For this review, take the finished solid that the model builds, in its own axes (mm). Face numbers are marked on the shaded views. A direction names the side the tool comes from. Give positions to 0.01 mm unless a question says otherwise; leave off trailing zeros. Order: outer loops, then holes, each group sorted by start corner. A loop starts at its lowest first (then second) coordinate and runs counter-clockwise, first axis right, second up. Notation, with made-up numbers: (83.5, 36.5) -> (116.5, 36.5) arc R6 ccw to (116.5, 45.5) -> close; hole circle Ø7 at (36, 51). An arc over 180 degrees is marked (long way). Use CSV: the item, a comma, the result in double quotes. Start each with the question number.
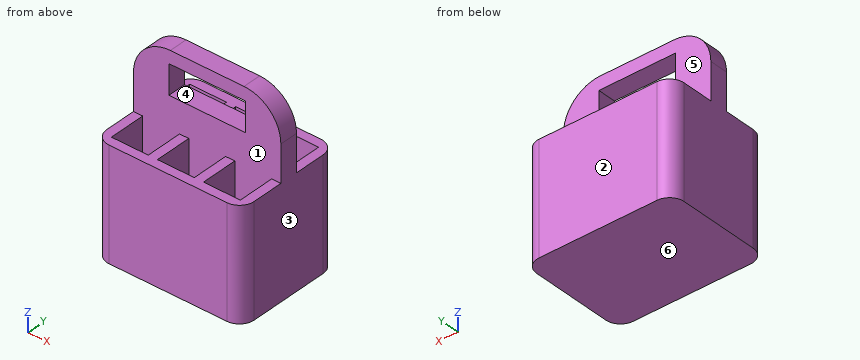
```python
from build123d import *

# Parameters (mm, degrees)
F0_W          = 3.175
F0_H          = 0.018239446
F0_H_2        = 12.681760554
F1_DEPTH      = 25.4
F2_R          = 6.35
F3_W          = 13.208
F3_H          = 5.08
F4_DEPTH      = 12.7
F5_W          = 6.35
F5_H          = 6.35
F6_DEPTH      = 4.7498
F6_DEPTH_BACK = 50.8
F7_R          = 2.54


with BuildPart() as f1:
    # F0 (on Right) → F1 (new body)
    with BuildSketch(Plane.YZ):
        Polygon((9.525, -9.525), (9.525, 9.525), (1.5875, 9.525), (1.5875, 9.506760554), (-1.5875, 9.506760554), (-1.5875, 9.525), (-9.525, 9.525), (-9.525, -9.525), align=None)
        with Locations((0, 9.515880277)):
            Rectangle(F0_W, F0_H)
        with Locations((0, 15.865880277)):
            Rectangle(F0_W, F0_H_2)
    extrude(amount=F1_DEPTH)

    # F2
    f2_edges = [f1.edges().sort_by_distance(p)[0] for p in [
        (25.4, 0, 22.206761),
        (0, 0, 22.206761),
    ]]
    fillet(f2_edges, radius=F2_R)

    # F3 (on Front) → F4 (cut, symmetric)
    with BuildSketch(Plane.XZ):
        with Locations((12.7, 17.4384163693)):
            Rectangle(F3_W, F3_H)
    extrude(amount=F4_DEPTH, both=True, mode=Mode.SUBTRACT)

    # F5 (on Top) → F6 (cut, two sides)
    with BuildSketch(Plane.XY) as f6_sk:
        with Locations((4.7625, 4.7625)):
            Rectangle(F5_W, F5_H)
        with Locations((20.6375, 4.7625)):
            Rectangle(F5_W, F5_H)
        with Locations((12.7, 4.7625)):
            Rectangle(F5_W, F5_H)
        with Locations((4.7625, -4.7625)):
            Rectangle(F5_W, F5_H)
        with Locations((12.7, -4.7625)):
            Rectangle(F5_W, F5_H)
        with Locations((20.6375, -4.7625)):
            Rectangle(F5_W, F5_H)
    extrude(amount=-F6_DEPTH, mode=Mode.SUBTRACT)
    extrude(f6_sk.sketch, amount=F6_DEPTH_BACK, mode=Mode.SUBTRACT)

    # F7
    f7_edges = [f1.edges().sort_by_distance(p)[0] for p in [
        (25.4, -9.525, 0),
        (0, -9.525, 0),
        (25.4, 9.525, 0),
        (0, 9.525, 0),
    ]]
    fillet(f7_edges, radius=F7_R)


solid = f1.part
```
1. Consider section D-D (y = -2.25). State the section outline as (x, z) points (1 decimal), plus the area to 3 significant figures.
2. Consider section C-C (z = 5.5). State how many separate pieces and enclosed holes the cut face has, plus the area to 3 significant figures.
3. For the marked faces 4, 5 and 6, list the 3-axis set-ups (+Z, -Z, +X, -X, +Y, -Y) from which the entire face can be reached by the end or side of a thin tool; tool diameter is ignored.
4. To check wall thickness, follow L1, parallel to Y at x = 5.25, z = 3 (1 decimal); L2, parallel to X at y = 4.25, z = 8 (1 decimal); L3, parallel to Z at x = 14.5, y = 0.5 (3 decimals). State the ranges of each line that lie inside material, in increasing order. Write a range as [from, to].
5. Consider section A-A (x = 16.25). State the section outline as (y, z) points (1 decimal), plus the area to 3 significant figures.
6. Clearance check with flat-ended pins moving along their axes: P1, Ø7, axis at x = 12, y = -3.5, coming from the +Z side; P2, Ø3, axis at x = 12.5, y = 3.5, coming from the +Z side; P3, Ø4, axis at x = 8, y = 6, coming from the +Z side (3 decimals). State where each tip first meets the part, or that it passes through.
7. Draft analysis for pull direction Y (two halves, no side actions). For the marked faces 1, 2 and 3, state which applies: +Y half, -Y half, draft (parallel to the pull), parting line (faces both ways), or undercut.
8. Consider section B-B (y = 0.25). State the section outline as (x, z) points (3 decimals).
Answer list:
1,outline,"(0, -9.5) -> (25.4, -9.5) -> (25.4, 9.5) -> (23.8, 9.5) -> (23.8, -4.7) -> (17.5, -4.7) -> (17.5, 9.5) -> (15.9, 9.5) -> (15.9, -4.7) -> (9.5, -4.7) -> (9.5, 9.5) -> (7.9, 9.5) -> (7.9, -4.7) -> (1.6, -4.7) -> (1.6, 9.5) -> (0, 9.5) -> close"
1,area,"212 mm2"
2,separate pieces,"1"
2,enclosed holes,"6"
2,area,"236 mm2"
3,face 4,"+Y, -Y"
3,face 5,"+Z"
3,face 6,"-Z, +X, -X, +Y, -Y"
4,L1,"[-9.5, -7.9], [-1.6, 1.6], [7.9, 9.5]"
4,L2,"[0, 1.6], [7.9, 9.5], [15.9, 17.5], [23.8, 25.4]"
4,L3,"[-9.525, 14.898], [19.978, 22.207]"
5,outline,"(-9.5, -9.5) -> (9.5, -9.5) -> (9.5, 9.5) -> (1.6, 9.5) -> (1.6, 14.9) -> (-1.6, 14.9) -> (-1.6, 9.5) -> (-9.5, 9.5) -> close; (-1.6, 20) -> (1.6, 20) -> (1.6, 22.2) -> (-1.6, 22.2) -> close"
5,area,"387 mm2"
6,P1,"z = 22.21"
6,P2,"z = -4.75"
6,P3,"z = 9.525"
7,face 1,"undercut"
7,face 2,"+Y half"
7,face 3,"draft"
8,outline,"(0, -9.525) -> (25.4, -9.525) -> (25.4, 15.857) arc R6.35 ccw to (19.05, 22.207) -> (6.35, 22.207) arc R6.35 ccw to (0, 15.857) -> close; hole (6.096, 14.898) -> (19.304, 14.898) -> (19.304, 19.978) -> (6.096, 19.978) -> close"
